from build123d import *

# Parameters (mm, degrees)
F1_DEPTH = 1.5
F2_W     = 12
F2_H     = 3.15
F3_DEPTH = 1.5
F5_DEPTH = 1.5
F7_DEPTH = 37.875
F8_DEPTH = 62


with BuildPart() as f1:
    # F0 (on Top) → F1 (new body)
    with BuildSketch(Plane.XY):
        Polygon((0, -34.35), (0, 34.35), (-55, 31.225), (-55, -31.225), align=None)
    extrude(amount=-F1_DEPTH)

    # F2 (on face) → F3 (cut, through all)
    with BuildSketch(Plane.XY):
        with Locations((-6, 13.425)):
            Rectangle(F2_W, F2_H)
        with Locations((-6, -13.425)):
            Rectangle(F2_W, F2_H)
    extrude(amount=-F3_DEPTH, mode=Mode.SUBTRACT)

    # F4 (on Top) → F5 (join, through all)
    with BuildSketch(Plane.XY):
        Polygon((-55, -29.25), (-55, 29.25), (-56.45, 26.25), (-56.45, -26.25), align=None)
    extrude(amount=-F5_DEPTH)

    # F6 (on Front) → F7 (join, symmetric)
    with BuildSketch(Plane.XZ):
        with BuildLine():
            ThreePointArc((-91.5, 0), (-70.5, 21), (-49.5, 0))
            Line((-49.5, 0), (-47.5, 0))
            ThreePointArc((-47.5, 0), (-70.5, 23), (-93.5, 0))
            Line((-93.5, 0), (-91.5, 0))
        make_face()
    extrude(amount=F7_DEPTH, both=True)

    # F7_face (on face) → F8 (cut)
    with BuildSketch(Plane(origin=(-70.5, 37.875, 14.015281), x_dir=(1, 0, 0), z_dir=(0, 1, 0))):
        with BuildLine():
            Line((-21, 14.015281), (-23, 14.015281))
            ThreePointArc((-23, 14.015281), (0, -8.984719), (23, 14.015281))
            Line((23, 14.015281), (21, 14.015281))
            ThreePointArc((21, 14.015281), (0, -6.984719), (-21, 14.015281))
        make_face()
    extrude(amount=-F8_DEPTH, mode=Mode.SUBTRACT)


solid = f1.part
Source: CAD feature listing. Evaluate the final solid. Frame: model axes, mm. A direction names the side the tool comes from. Coordinates: 2 decimals unless noted, no trailing zeros. Loops run counter-clockwise (first coordinate to the right, second up) from the corner with the lowest first, then second, coordinate; pieces in that order, holes last. Notation, with made-up numbers: (7.5, 43.25) -> (55.5, 43.25) arc R14 cw to (55.5, 57.25) -> close; hole circle Ø4 at (18, 24). An arc over 180 degrees is marked (long way). Answer in a Markdown table with one row per item. Add a question column.
Q1. Section C-C on y = -14. Return the cut outline in (x, z).
Q2. Pull-direction query (Z, two-part tool) for faces 1 (the face through (-49, -35, 0)), 2 (the face through (-70.962, -31.096, 20.995)), 3 (the face through (-74, -37.875, 21)), 4 (the face through (-69.994, -31.096, 22.994)); classes: pulls with the +Z half, pulls with the -Z half, needs draft (parallel to the pull), parting line crosses it, or undercut.
Q3. Section B-B on x = -6. Return the cut outline in (y, z), and give its area (3 significant figures).
Q4. Section A-A on z = 3. Return the cut outline in (x, y) (1 decimal).
Q5. Ray query, line 1 along Y through (x, z) = (-72, 21.75) (3 decimals); line 2 along Z through (x, y) = (-17, -24.5); line 3 along X through (y, z) = (-29, 18). Return the intervals inside material, ascending.
Q6. Section D-D on x = -70.5. Return the cut outline in (y, z) (3 decimals), and give its area (3 significant figures).
Q7. Reachability of faces 5 (the face through (-29, 0, -1.5)), 6 (the face through (-93, -31, 0)), 7 (the face through (-74, -24.125, 21)) from +Z, -Z, +X, -X, +Y, -Y: full face, straight path, thin tool, end or side. Return the list, or none.
Q8. Contact query for flat-ended pins moving along their axis: pin 1 Ø1.6 at (x, y) = (-92.5, -32.5) entering from -Z; pin 2 Ø0.8 at (x, z) = (-8, -1) entering from -Y; pin 3 Ø8 at (y, z) = (-28, 11.5) entering from -X. Output: stop coordinate, or through.
Computed values:
| question | item | result |
|---|---|---|
| 1 | outline | (-56.45, -1.5) -> (-12, -1.5) -> (-12, 0) -> (-56.45, 0) -> close |
| 2 | face 1 | pulls with the -Z half |
| 2 | face 2 | undercut |
| 2 | face 3 | needs draft |
| 2 | face 4 | pulls with the +Z half |
| 3 | outline | (-34.01, -1.5) -> (-15, -1.5) -> (-15, 0) -> (-34.01, 0) -> close; (-11.85, -1.5) -> (11.85, -1.5) -> (11.85, 0) -> (-11.85, 0) -> close; (15, -1.5) -> (34.01, -1.5) -> (34.01, 0) -> (15, 0) -> close |
| 3 | area | 92.6 mm^2 |
| 4 | outline | (-93.3, -37.9) -> (-91.3, -37.9) -> (-91.3, -24.1) -> (-93.3, -24.1) -> close; (-49.7, -37.9) -> (-47.7, -37.9) -> (-47.7, -24.1) -> (-49.7, -24.1) -> close |
| 5 | line 1 | y = -37.875 to -24.125 |
| 5 | line 2 | z = -1.5 to 0 |
| 5 | line 3 | x = -84.82 to -81.32, -59.68 to -56.18 |
| 6 | outline | (-37.875, 21) -> (-24.125, 21) -> (-24.125, 23) -> (-37.875, 23) -> close |
| 6 | area | 27.5 mm^2 |
| 7 | face 5 | -Z, +X, -X, +Y, -Y |
| 7 | face 6 | -Z, -X, +Y, -Y |
| 7 | face 7 | +Z, +X, -X, +Y |
| 8 | pin 1 | stops at z = 0 |
| 8 | pin 2 | stops at y = -33.92 |
| 8 | pin 3 | stops at x = -92.24 |
